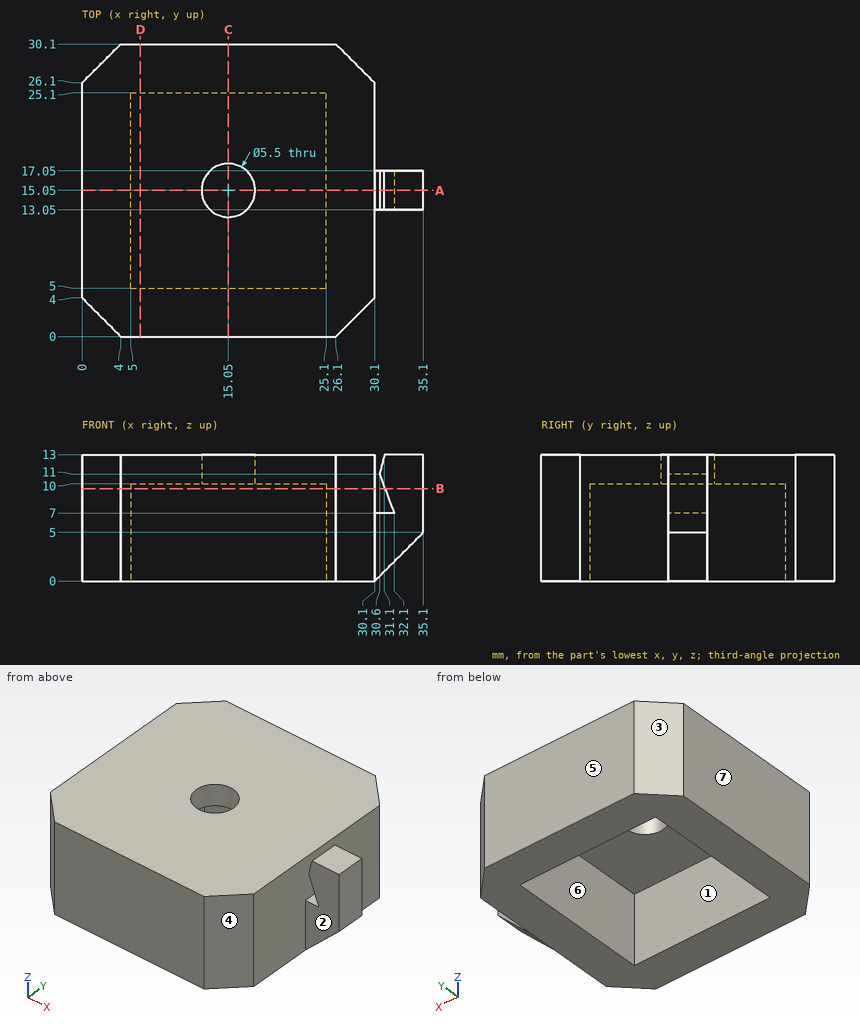
Could you check a few things on this drawing? It's one solid part, dimensions in mm from its lowest x, y, z. A direction names the side the tool comes from. Coordinates: 2 decimals unless noted, no trailing zeros. Order: outer loops, then holes, each group sorted by start corner. A loop starts at its lowest first (then second) coordinate and runs counter-clockwise, first axis right, second up. Notation, with made-up numbers: (-19.5, 62.5) - (39.5, 62.5) arc R33 ccw to (39.5, 97.5) - close; hole circle Ø8 at (71, 11). An arc over 180 degrees is marked (long way). One line per question, with ' | ' between items.
(1) For the marked faces 1, 2 and 3, which set-ups out of +Z, -Z, +X, -X, +Y, -Y let a thin tool reach every point of the face, with its end or its side?
Report:
face 1: -Z | face 2: +Z, -Z, +X, -Y | face 3: +Z, -Z, -X, +Y
(2) Suppose I cut it at B-B on z = 9.5. List the corners of the cut face in (x, y) for me, and give its area (3 significant figures).
Report:
outline: (0, 4) - (4, 0) - (26.1, 0) - (30.1, 4) - (30.1, 26.1) - (26.1, 30.1) - (4, 30.1) - (0, 26.1) - close; (31.16, 13.05) - (35.1, 13.05) - (35.1, 17.05) - (31.16, 17.05) - close; hole (5, 5) - (25.1, 5) - (25.1, 25.1) - (5, 25.1) - close | area: 486 mm2
(3) Suppose I cut it at D-D on x = 6. List the corners of the cut face in (y, z) for me, and give its area (3 significant figures).
Report:
outline: (0, 0) - (5, 0) - (5, 10) - (25.1, 10) - (25.1, 0) - (30.1, 0) - (30.1, 13) - (0, 13) - close | area: 190 mm2
(4) Suppose I cut it at C-C on x = 15.05. List the corners of the cut face in (y, z) for me.
Report:
outline: (0, 0) - (5, 0) - (5, 10) - (12.3, 10) - (12.3, 13) - (0, 13) - close; (17.8, 10) - (25.1, 10) - (25.1, 0) - (30.1, 0) - (30.1, 13) - (17.8, 13) - close
(5) If we mould it in two halves opening along X, with no side actions, what happens to the marked faces 4, 5, 6 and 7? For each: pulls with the +X half, pulls with the -X half, needs draft (parallel to the pull), parting line crosses it, or undercut.
Report:
face 4: pulls with the +X half | face 5: needs draft | face 6: undercut | face 7: pulls with the -X half
(6) Will these pins go through, and if not, where does the flat tip stop? pin 1 (2.5 mm diameter, centred on x = 33.5, z = 8, fed in from -Y); pin 2 (7 mm diameter, centred on x = 15.05, y = 15.05, fed in from -Z); pin 3 (5.5 mm diameter, centred on x = 33, z = 7.5, fed in from +Y).
Report:
pin 1: stops at y = 13.05 | pin 2: stops at z = 10 | pin 3: stops at y = 17.05
(7) Suppose I cut it at A-A on y = 15.05. List the corners of the cut face in (x, z) for me.
Report:
outline: (0, 0) - (5, 0) - (5, 10) - (12.3, 10) - (12.3, 13) - (0, 13) - close; (17.8, 10) - (25.1, 10) - (25.1, 0) - (30.1, 0) - (35.1, 5) - (35.1, 13) - (31.1, 13) - (30.6, 11) - (32.1, 7) - (30.1, 7) - (30.1, 13) - (17.8, 13) - close
(8) If I drill on L1, parallel to Y at x = 6.5, z = 1.75; L2, parallel to Y at x = 15.05, z = 11.6; L3, parallel to Z at x = 5.5, y = 10.5, over which ranges is the centre line in solid material (lowest first)?
Report:
L1: y = 0 to 5, 25.1 to 30.1 | L2: y = 0 to 12.3, 17.8 to 30.1 | L3: z = 10 to 13
